```python
from build123d import *

# Parameters (mm, degrees)
SKETCH2_W             = 100
SKETCH2_H             = 17
BASE_DEPTH            = 2
M3_CLEARANCE_HOLE1_D  = 3.4
M4X0_7_TAPPED_HOLE1_D = 3.3
SKETCH9_W             = 18.2
SKETCH9_H             = 9
CUT_EXTRUDE1_DEPTH    = 10
FILLET3_R             = 4


with BuildPart() as part:
    # Sketch2 → Base (new body, symmetric)
    with BuildSketch(Plane.XY):
        with Locations((0, 8.5)):
            Rectangle(SKETCH2_W, SKETCH2_H)
    extrude(amount=BASE_DEPTH, both=True)

    # M3 Clearance Hole1 (through all)
    with Locations(Plane(origin=(0, 4, -2), x_dir=(1, 0, 0), z_dir=(0, 0, -1))):
        with Locations((-8, 0), (8, 0)):
            Hole(M3_CLEARANCE_HOLE1_D / 2)

    # M4x0.7 Tapped Hole1 (through all)
    with Locations(Plane(origin=(0, 0, -2), x_dir=(-1, 0, 0), z_dir=(0, 0, -1))):
        with Locations((-45.8, 13), (45.8, 13)):
            Hole(M4X0_7_TAPPED_HOLE1_D / 2)

    # Sketch9 → Cut-Extrude1 (cut)
    with BuildSketch(Plane(origin=(0, 0, -2), x_dir=(-1, 0, 0), z_dir=(0, 0, -1))):
        with Locations((40.9, 4.5)):
            Rectangle(SKETCH9_W, SKETCH9_H)
        with Locations((-40.9, 4.5)):
            Rectangle(SKETCH9_W, SKETCH9_H)
    extrude(amount=-CUT_EXTRUDE1_DEPTH, mode=Mode.SUBTRACT)

    # Fillet3
    fillet3_edges = [part.edges().sort_by_distance(p)[0] for p in [
        (-31.8, 9, 0),
        (-50, 9, 0),
        (50, 9, 0),
        (31.8, 9, 0),
    ]]
    fillet(fillet3_edges, radius=FILLET3_R)


solid = part.part
```
Input: part model. Units: mm. Frame: model coordinates. A direction names the side the tool comes from. Round coordinates to 2 decimals unless told otherwise and drop trailing zeros. Loops run counter-clockwise (first coordinate to the right, second up) from the corner with the lowest first, then second, coordinate; pieces in that order, holes last. Notation, with made-up numbers: (-37.5, 64) - (-32.5, 64) arc R14 ccw to (-32.5, 72) - close; hole circle Ø9 at (6.25, 9.5). An arc over 180 degrees is marked (long way). One line per item, written item: value. Start each with the question number.
(1) Section A-A, the plane y = 4. Return loops of the section in (x, z).
(2) Contact query for flat-ended pins moving along their axis: P1, Ø2, axis at x = 42, z = -0.5, coming from the -Y side; P2, Ø2, axis at y = 3.5, z = 0, coming from the -X side. Output: stop coordinate, or through.
(3) Section B-B, the plane z = 0.7. Return loops of the section in (x, y).
(4) Access query for faces 1 (the flat face through (-31.8, 2, 0)), 2 (the flat face through (50, 15, 0)), 3 (the flat face through (41, 9, 0)). Directions: +Z, -Z, +X, -X, +Y, -Y. A direction counts if a zero-diameter tool reaches every point of the face in a straight line with its end or side. Return the directions, or none.
(5) Section C-C, the plane x = -8. Return loops of the section in (y, z).
(6) Draft query along Y for faces 4 (the flat face through (-50, 15, 0)), 5 (the cylindrical face through (47.324, 12.368, 0.028)), 6 (the flat face through (-41, 9, 0)). Return one class per face: +Y half, -Y half, draft (parallel to the pull), parting line (faces both ways), or undercut.
(7) Ray query, line 1 (X direction, y = 4, z = 1.3); line 2 (Y direction, x = 8, z = 0.3); line 3 (Y direction, x = -45.8, z = 0.4). Return the intervals inside material, ascending. Write a range as [from, to].
Results below:
1. outline: (-31.8, -2) - (-9.7, -2) - (-9.7, 2) - (-31.8, 2) - close; (-6.3, -2) - (6.3, -2) - (6.3, 2) - (-6.3, 2) - close; (9.7, -2) - (31.8, -2) - (31.8, 2) - (9.7, 2) - close
2. P1: y = 9
2. P2: x = -31.8
3. outline: (-50, 13) arc R4 ccw to (-46, 9) - (-35.8, 9) arc R4 cw to (-31.8, 5) - (-31.8, 0) - (31.8, 0) - (31.8, 5) arc R4 cw to (35.8, 9) - (46, 9) arc R4 ccw to (50, 13) - (50, 17) - (-50, 17) - close; hole circle Ø3.3 at (-45.8, 13); hole circle Ø3.4 at (-8, 4); hole circle Ø3.4 at (8, 4); hole circle Ø3.3 at (45.8, 13)
4. face 1: +Z, -Z, -X, -Y
4. face 2: +Z, -Z, +X, +Y, -Y
4. face 3: +Z, -Z, +X, -Y
5. outline: (0, -2) - (2.3, -2) - (2.3, 2) - (0, 2) - close; (5.7, -2) - (17, -2) - (17, 2) - (5.7, 2) - close
6. face 4: draft
6. face 5: undercut
6. face 6: -Y half
7. line 1: [-31.8, -9.7], [-6.3, 6.3], [9.7, 31.8]
7. line 2: [0, 2.3], [5.7, 17]
7. line 3: [9, 11.35], [14.65, 17]
